```python
from build123d import *

# Parameters (mm, degrees)
SKETCH1_R           = 68
BOSS_EXTRUDE3_DEPTH = 23
BOSS_EXTRUDE4_START = -3
SKETCH1_6_R         = 68
SKETCH1_6_R_2       = 12
BOSS_EXTRUDE4_DEPTH = 3


with BuildPart() as part:
    # Sketch1 → Boss-Extrude3 (new body)
    with BuildSketch(Plane(origin=(0, 0, 0), x_dir=(1, 0, 0), z_dir=(0, 1, 0))):
        with Locations(Location((0, 0, 0), (0, 0, 270))):
            Circle(SKETCH1_R)
        with BuildLine():
            ThreePointArc((3.63159136, 62.176765992), (12.15075821, 61.085986608), (20.438865295, 58.833591344))
            ThreePointArc((20.438865295, 58.833591344), (21.621613929, 52.199193587), (27.149171151, 56.054091651))
            ThreePointArc((27.149171151, 56.054091651), (34.602431839, 51.786198893), (41.397689987, 46.533535742))
            ThreePointArc((41.397689987, 46.533535742), (39.951533137, 39.951533137), (46.533535742, 41.397689987))
            ThreePointArc((46.533535742, 41.397689987), (51.786198893, 34.602431839), (56.054091651, 27.149171151))
            ThreePointArc((56.054091651, 27.149171151), (52.199193587, 21.621613929), (58.833591344, 20.438865295))
            ThreePointArc((58.833591344, 20.438865295), (61.085986608, 12.15075821), (62.176765992, 3.63159136))
            ThreePointArc((62.176765992, 3.63159136), (56.5, 0), (62.176765992, -3.63159136))
            ThreePointArc((62.176765992, -3.63159136), (61.085986608, -12.15075821), (58.833591344, -20.438865295))
            ThreePointArc((58.833591344, -20.438865295), (52.199193587, -21.621613929), (56.054091651, -27.149171151))
            ThreePointArc((56.054091651, -27.149171151), (51.786198893, -34.602431839), (46.533535742, -41.397689987))
            ThreePointArc((46.533535742, -41.397689987), (39.951533137, -39.951533137), (41.397689987, -46.533535742))
            ThreePointArc((41.397689987, -46.533535742), (34.602431839, -51.786198893), (27.149171151, -56.054091651))
            ThreePointArc((27.149171151, -56.054091651), (21.621613929, -52.199193587), (20.438865295, -58.833591344))
            ThreePointArc((20.438865295, -58.833591344), (12.15075821, -61.085986608), (3.631591361, -62.176765992))
            ThreePointArc((3.631591361, -62.176765992), (0, -56.5), (-3.63159136, -62.176765992))
            ThreePointArc((-3.63159136, -62.176765992), (-12.15075821, -61.085986608), (-20.438865295, -58.833591344))
            ThreePointArc((-20.438865295, -58.833591344), (-21.621613929, -52.199193587), (-27.149171151, -56.054091651))
            ThreePointArc((-27.149171151, -56.054091651), (-34.602431839, -51.786198893), (-41.397689987, -46.533535742))
            ThreePointArc((-41.397689987, -46.533535742), (-39.951533137, -39.951533137), (-46.533535742, -41.397689987))
            ThreePointArc((-46.533535742, -41.397689987), (-51.786198893, -34.602431839), (-56.054091651, -27.149171151))
            ThreePointArc((-56.054091651, -27.149171151), (-52.199193587, -21.621613929), (-58.833591344, -20.438865295))
            ThreePointArc((-58.833591344, -20.438865295), (-61.085986608, -12.15075821), (-62.176765992, -3.63159136))
            ThreePointArc((-62.176765992, -3.63159136), (-56.5, 0), (-62.176765992, 3.63159136))
            ThreePointArc((-62.176765992, 3.63159136), (-61.085986608, 12.15075821), (-58.833591344, 20.438865295))
            ThreePointArc((-58.833591344, 20.438865295), (-52.199193587, 21.621613929), (-56.054091651, 27.149171151))
            ThreePointArc((-56.054091651, 27.149171151), (-51.786198893, 34.602431839), (-46.533535742, 41.397689987))
            ThreePointArc((-46.533535742, 41.397689987), (-39.951533137, 39.951533137), (-41.397689987, 46.533535742))
            ThreePointArc((-41.397689987, 46.533535742), (-34.602431839, 51.786198893), (-27.149171151, 56.054091651))
            ThreePointArc((-27.149171151, 56.054091651), (-21.621613929, 52.199193587), (-20.438865295, 58.833591344))
            ThreePointArc((-20.438865295, 58.833591344), (-12.15075821, 61.085986608), (-3.63159136, 62.176765992))
            ThreePointArc((-3.63159136, 62.176765992), (0, 56.5), (3.63159136, 62.176765992))
        make_face(mode=Mode.SUBTRACT)
    extrude(amount=BOSS_EXTRUDE3_DEPTH)

    # Sketch1_6 → Boss-Extrude4 (add)
    with BuildSketch(Plane(origin=(0, 0, 0), x_dir=(1, 0, 0), z_dir=(0, 1, 0)).offset(BOSS_EXTRUDE4_START)):
        with Locations(Location((0, 0, 0), (0, 0, 270))):
            Circle(SKETCH1_6_R)
        with Locations(Location((0, 0, 0), (0, 0, 270))):
            Circle(SKETCH1_6_R_2, mode=Mode.SUBTRACT)
    extrude(amount=BOSS_EXTRUDE4_DEPTH)


solid = part.part
```
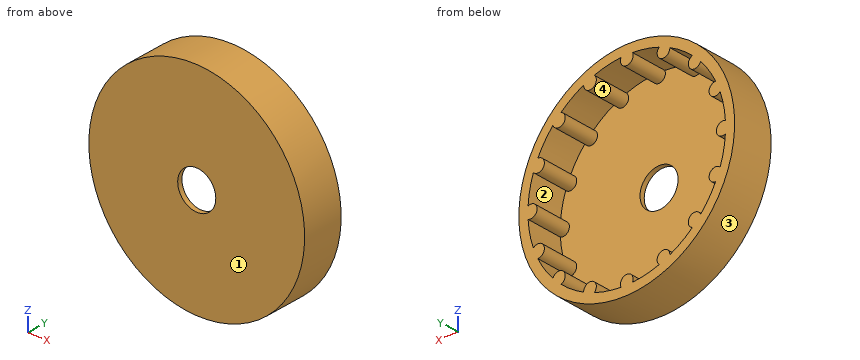
Here's how the part is built. I have some questions about the finished solid (model axes, mm). Face numbers are marked on the shaded views. Round coordinates to 2 decimals unless told otherwise and drop trailing zeros. Loops run counter-clockwise (first coordinate to the right, second up) from the corner with the lowest first, then second, coordinate; pieces in that order, holes last. Notation, with made-up numbers: (-11.5, 33.25) -> (-0.5, 33.25) arc R12 ccw to (-0.5, 51.25) -> close; hole circle Ø9 at (45, 34). An arc over 180 degrees is marked (long way). Answer as CSV lines item,"result". Start each with the question number.
1. Imagine slicing it at A-A on x = 0. Write out the boundary of the cut face in (y, z), plus the area to 3 significant figures.
2. If we mould it in two halves opening along X, with no side actions, what happens to the marked faces 1, 2, 3 and 4? For each: pulls with the +X half, pulls with the -X half, needs draft (parallel to the pull), parting line crosses it, or undercut.
3. Imagine slicing it at D-D on z = 60.5. Write out the boundary of the cut face in (x, y), plus the area to 3 significant figures.
4. I'm going to push flat-ended pins straight in: P1, Ø4, axis at x = 32, z = -48.5, coming from the +Y side; P2, Ø12, axis at x = -30, y = 19.5, coming from the -Z side; P3, Ø6, axis at y = 9.5, z = -14, coming from the +X side. Where does each tip first touch, or does it pass through?
5. Imagine slicing it at B-B on z = 0. Write out the boundary of the cut face in (x, y), plus the area to 3 significant figures.
6. I need wall thicknesses on probe 1 along X at (y, z) = (-2.35, 0); probe 2 along X at (y, z) = (16.25, -55); probe 3 along Y at (x, z) = (-49.5, 1). Which ranges of each line are inside material? Lowest first, please. Write a range as from..to.
Solution:
1,outline,"(-3, -68) -> (23, -68) -> (23, -56.5) -> (0, -56.5) -> (0, -12) -> (-3, -12) -> close; (-3, 12) -> (0, 12) -> (0, 56.5) -> (23, 56.5) -> (23, 68) -> (-3, 68) -> close"
1,area,"865 mm²"
2,face 1,"needs draft"
2,face 2,"undercut"
2,face 3,"parting line crosses it"
2,face 4,"undercut"
3,outline,"(-31.04, -3) -> (31.04, -3) -> (31.04, 23) -> (14.79, 23) -> (14.79, 0) -> (4, 0) -> (4, 23) -> (-4, 23) -> (-4, 0) -> (-14.79, 0) -> (-14.79, 23) -> (-31.04, 23) -> close"
3,area,"1,120 mm²"
4,P1,"y = 0"
4,P2,"z = -63.62"
4,P3,"x = 67.1"
5,outline,"(-68, -3) -> (-12, -3) -> (-12, 0) -> (-56.5, 0) -> (-56.5, 23) -> (-68, 23) -> close; (12, -3) -> (68, -3) -> (68, 23) -> (56.5, 23) -> (56.5, 0) -> (12, 0) -> close"
5,area,"865 mm²"
6,probe 1,"-68..-12, 12..68"
6,probe 2,"-39.99..-29.23, -27.05..-19.25, 19.25..27.05, 29.23..39.99"
6,probe 3,"-3..0"
